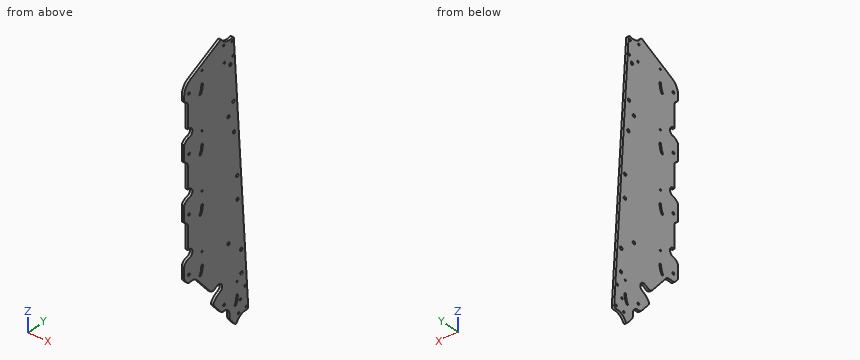
from build123d import *

# Parameters (mm, degrees)
SKETCH_1_R      = 2.5
SKETCH_1_R_2    = 1.6
SKETCH_1_R_3    = 1.3
SKETCH_1_R_4    = 1.9
EXTRUDE_1_DEPTH = 4


with BuildPart() as part:
    # 草图1 → 凸台-拉伸1 (new body)
    with BuildSketch(Plane.ZY):
        with BuildLine():
            Line((79.941847196, 312.779286974), (79.941847196, 310.37938842))
            Line((79.941847196, 310.37938842), (118.048778684, 310.37938842))
            ThreePointArc((118.048778684, 310.37938842), (121.212295154, 309.477639448), (123.424912382, 307.043442935))
            ThreePointArc((123.424912382, 307.043442935), (123.908451597, 306.156590075), (124.459804418, 305.310228312))
            ThreePointArc((124.459804418, 305.310228312), (126.599767036, 303.449448704), (129.355274977, 302.779286974))
            Line((129.355274977, 302.779286974), (135.846674735, 302.779286974))
            ThreePointArc((135.846674735, 302.779286974), (147.714917725, 306.255118752), (155.832977431, 315.5843044))
            Line((155.832977431, 315.5843044), (184.100349844, 377.02653737))
            ThreePointArc((184.100349844, 377.02653737), (184.25423495, 379.122829036), (182.994670387, 380.805569803))
            ThreePointArc((182.994670387, 380.805569803), (175.575423742, 390.035917566), (175.217785471, 401.873004854))
            ThreePointArc((175.217785471, 401.873004854), (174.813539386, 404.446095635), (172.549129806, 405.733208807))
            Line((172.549129806, 405.733208807), (-265.913463366, 435.515010668))
            ThreePointArc((-265.913463366, 435.515010668), (-268.349260645, 434.525893618), (-269.070634733, 431.997835004))
            ThreePointArc((-269.070634733, 431.997835004), (-270.458967767, 420.871071163), (-277.882819523, 412.467573839))
            ThreePointArc((-277.882819523, 412.467573839), (-279.312515533, 410.13392022), (-278.252765969, 407.610648385))
            Line((-278.252765969, 407.610648385), (-268.246230566, 399.190213281))
            ThreePointArc((-268.246230566, 399.190213281), (-265.544431584, 397.566061892), (-262.471282959, 396.863678095))
            Line((-262.471282959, 396.863678095), (-255.629318556, 396.408593428))
            ThreePointArc((-255.629318556, 396.408593428), (-248.6530075, 392.882824378), (-246.344722675, 385.41477346))
            ThreePointArc((-246.344722675, 385.41477346), (-245.547224173, 381.106497376), (-242.780709967, 377.708903254))
            Line((-242.780709967, 377.708903254), (-225.96618646, 363.559589999))
            ThreePointArc((-225.96618646, 363.559589999), (-224.259021966, 363.148943594), (-222.527086507, 363.437804541))
            ThreePointArc((-222.527086507, 363.437804541), (-216.093640019, 369.198004343), (-211.901591148, 376.74756471))
            ThreePointArc((-211.901591148, 376.74756471), (-202.96771311, 381.012048641), (-198.703229179, 372.078170603))
            ThreePointArc((-198.703229179, 372.078170603), (-199.907426668, 369.068297365), (-201.351406018, 366.165823913))
            ThreePointArc((-201.351406018, 366.165823913), (-202.203284687, 360.847165515), (-199.49001514, 356.193995329))
            Line((-199.49001514, 356.193995329), (-166.466058225, 328.404548243))
            ThreePointArc((-166.466058225, 328.404548243), (-163.838636178, 324.972953793), (-162.904676824, 320.753130691))
            Line((-162.904676824, 320.753130691), (-162.904676824, 314.217366152))
            ThreePointArc((-162.904676824, 314.217366152), (-162.15750934, 310.841507671), (-160.055571702, 308.096232111))
            Line((-160.055571702, 308.096232111), (-156.52807865, 305.127869423))
            ThreePointArc((-156.52807865, 305.127869423), (-153.516253341, 303.384762625), (-150.089460052, 302.779286974))
            Line((-150.089460052, 302.779286974), (-132.962822931, 302.779286974))
            ThreePointArc((-132.962822931, 302.779286974), (-131.057359543, 303.089892518), (-129.349178653, 303.989550548))
            ThreePointArc((-129.349178653, 303.989550548), (-127.378799895, 305.843763559), (-125.854682643, 308.079286974))
            ThreePointArc((-125.854682643, 308.079286974), (-124.70730834, 310.334067306), (-124.058152804, 312.779286974))
            ThreePointArc((-124.058152804, 312.779286974), (-117.058152804, 319.779286974), (-110.058152804, 312.779286974))
            Line((-110.058152804, 312.779286974), (-110.058152804, 310.375194841))
            Line((-110.058152804, 310.375194841), (-71.897768127, 310.375194841))
            ThreePointArc((-71.897768127, 310.375194841), (-68.768086545, 309.494285893), (-66.557393134, 307.110225907))
            ThreePointArc((-66.557393134, 307.110225907), (-65.945300527, 306.047683601), (-65.231544729, 305.050584724))
            ThreePointArc((-65.231544729, 305.050584724), (-63.141167069, 303.376870223), (-60.530823557, 302.779286974))
            Line((-60.530823557, 302.779286974), (-36.305637158, 302.779286974))
            ThreePointArc((-36.305637158, 302.779286974), (-33.16644373, 305.003787341), (-30.854682657, 308.079286974))
            ThreePointArc((-30.854682657, 308.079286974), (-29.707305648, 310.334074366), (-29.058150487, 312.779301913))
            ThreePointArc((-29.058150487, 312.779301913), (-22.058145334, 319.779284657), (-15.058155121, 312.779286974))
            Line((-15.058155121, 312.779286974), (-15.058155121, 310.354804619))
            Line((-15.058155121, 310.354804619), (23.075565874, 310.354804619))
            ThreePointArc((23.075565874, 310.354804619), (26.234507213, 309.455891721), (28.446910847, 307.028501158))
            ThreePointArc((28.446910847, 307.028501158), (28.930044794, 306.145924462), (29.48046838, 305.303669209))
            ThreePointArc((29.48046838, 305.303669209), (31.619349297, 303.447603066), (34.37128438, 302.779286974))
            Line((34.37128438, 302.779286974), (58.694362842, 302.779286974))
            ThreePointArc((58.694362842, 302.779286974), (61.833556273, 305.00378734), (64.14531735, 308.079286974))
            ThreePointArc((64.14531735, 308.079286974), (65.292691668, 310.334067319), (65.941847214, 312.779287004))
            ThreePointArc((65.941847214, 312.779287004), (72.94184722, 319.77928698), (79.941847196, 312.779286974))
        make_face()
        with Locations((134.697589837, 398.714435962)):
            Circle(SKETCH_1_R, mode=Mode.SUBTRACT)
        with Locations((-205.302410163, 421.329108832)):
            Circle(SKETCH_1_R, mode=Mode.SUBTRACT)
        with Locations((24.697589837, 406.030947773)):
            Circle(SKETCH_1_R, mode=Mode.SUBTRACT)
        with Locations((54.697589837, 394.714435962)):
            Circle(SKETCH_1_R, mode=Mode.SUBTRACT)
        with Locations((-145.302410163, 394.714435962)):
            Circle(SKETCH_1_R, mode=Mode.SUBTRACT)
        with Locations((-85.302410163, 413.347459584)):
            Circle(SKETCH_1_R, mode=Mode.SUBTRACT)
        with Locations((-229.912547558, 429.226877683)):
            Circle(SKETCH_1_R_2, mode=Mode.SUBTRACT)
        with Locations((-263.830685058, 431.584832)):
            Circle(SKETCH_1_R_2, mode=Mode.SUBTRACT)
        with Locations((-245.82758059, 419.331621378)):
            Circle(SKETCH_1_R_2, mode=Mode.SUBTRACT)
        with Locations((-213.924753581, 412.419296618)):
            Circle(SKETCH_1_R_3, mode=Mode.SUBTRACT)
        with Locations((-265.82758059, 415.709933316)):
            Circle(SKETCH_1_R_2, mode=Mode.SUBTRACT)
        with Locations((145.452321386, 404.165877908)):
            Circle(SKETCH_1_R_2, mode=Mode.SUBTRACT)
        with Locations((172.223627163, 384.384644706)):
            Circle(SKETCH_1_R_2, mode=Mode.SUBTRACT)
        with Locations((169.397149412, 402.539467503)):
            Circle(SKETCH_1_R_2, mode=Mode.SUBTRACT)
        with Locations((144.282792088, 386.203912503)):
            Circle(SKETCH_1_R_2, mode=Mode.SUBTRACT)
        with Locations((-236.412834805, 385.419296624)):
            Circle(SKETCH_1_R_4, mode=Mode.SUBTRACT)
        with Locations((-128.211318153, 339.779286974)):
            Circle(SKETCH_1_R_3, mode=Mode.SUBTRACT)
        with Locations((62, 339.779286968)):
            Circle(SKETCH_1_R_3, mode=Mode.SUBTRACT)
        with Locations((40, 312.779286974)):
            Circle(SKETCH_1_R_4, mode=Mode.SUBTRACT)
        with Locations((-47.3651173, 412.828527404)):
            Circle(SKETCH_1_R, mode=Mode.SUBTRACT)
        with Locations((-55.488081224, 312.779286974)):
            Circle(SKETCH_1_R_4, mode=Mode.SUBTRACT)
        with Locations((-33, 339.779286968)):
            Circle(SKETCH_1_R_3, mode=Mode.SUBTRACT)
        with Locations((-168.130178692, 420.86106375)):
            Circle(SKETCH_1_R, mode=Mode.SUBTRACT)
        with Locations((73.399944092, 404.795991058)):
            Circle(SKETCH_1_R, mode=Mode.SUBTRACT)
        with Locations((157, 339.779286968)):
            Circle(SKETCH_1_R_3, mode=Mode.SUBTRACT)
        with Locations((-150.058152804, 312.779286974)):
            Circle(SKETCH_1_R_4, mode=Mode.SUBTRACT)
        with Locations((135, 312.779286974)):
            Circle(SKETCH_1_R_4, mode=Mode.SUBTRACT)
        with BuildLine():
            ThreePointArc((-235.893747688, 414.018996163), (-243.357483185, 413.10813588), (-250.274012295, 410.158790343))
            ThreePointArc((-250.274012295, 410.158790343), (-250.815185629, 407.961716967), (-248.618112252, 407.420543633))
            ThreePointArc((-248.618112252, 407.420543633), (-242.527853555, 410.017551036), (-235.955759474, 410.819597073))
            ThreePointArc((-235.955759474, 410.819597073), (-234.325054036, 412.388290724), (-235.893747688, 414.018996163))
        make_face(mode=Mode.SUBTRACT)
        with BuildLine():
            ThreePointArc((-54.968994107, 341.378986513), (-62.432729604, 340.468126231), (-69.349258714, 337.518780694))
            ThreePointArc((-69.349258714, 337.518780694), (-69.890432048, 335.321707317), (-67.693358671, 334.780533983))
            ThreePointArc((-67.693358671, 334.780533983), (-61.603099974, 337.377541387), (-55.031005893, 338.179587423))
            ThreePointArc((-55.031005893, 338.179587423), (-53.400300455, 339.748281075), (-54.968994107, 341.378986513))
        make_face(mode=Mode.SUBTRACT)
        with BuildLine():
            ThreePointArc((-150.180312259, 341.378986519), (-157.644047756, 340.468126237), (-164.560576866, 337.5187807))
            ThreePointArc((-164.560576866, 337.5187807), (-165.1017502, 335.321707323), (-162.904676824, 334.780533989))
            ThreePointArc((-162.904676824, 334.780533989), (-156.814418127, 337.377541393), (-150.242324046, 338.179587429))
            ThreePointArc((-150.242324046, 338.179587429), (-148.611618608, 339.748281081), (-150.180312259, 341.378986519))
        make_face(mode=Mode.SUBTRACT)
        with BuildLine():
            ThreePointArc((40.031005893, 341.378986519), (32.567270396, 340.468126237), (25.650741286, 337.5187807))
            ThreePointArc((25.650741286, 337.5187807), (25.109567952, 335.321707323), (27.306641329, 334.780533989))
            ThreePointArc((27.306641329, 334.780533989), (33.396900026, 337.377541393), (39.968994107, 338.179587429))
            ThreePointArc((39.968994107, 338.179587429), (41.599699545, 339.748281081), (40.031005893, 341.378986519))
        make_face(mode=Mode.SUBTRACT)
        with BuildLine():
            ThreePointArc((135.031005893, 341.378986513), (127.567270396, 340.468126231), (120.650741287, 337.518780694))
            ThreePointArc((120.650741287, 337.518780694), (120.109567952, 335.321707317), (122.306641329, 334.780533983))
            ThreePointArc((122.306641329, 334.780533983), (128.396900026, 337.377541387), (134.968994107, 338.179587423))
            ThreePointArc((134.968994107, 338.179587423), (136.599699545, 339.748281075), (135.031005893, 341.378986513))
        make_face(mode=Mode.SUBTRACT)
    extrude(amount=EXTRUDE_1_DEPTH)


solid = part.part
Design review of the part built by this model. Coordinates are the model's own, in mm. Give positions to 0.01 mm unless a question says otherwise; leave off trailing zeros. Loops run counter-clockwise (first coordinate to the right, second up) from the corner with the lowest first, then second, coordinate; pieces in that order, holes last. Notation, with made-up numbers: M 31,47 L 80,47 A30 ccw 80,69 Z; hole C 70,31.25 d3. An arc over 180 degrees is marked long. One line per question, with ' | ' between items. Start each with the question number.
1. Insertion check: P1, Ø1, axis at x = -0.5, z = 64, coming from the +Y side; P2, Ø1.5, axis at x = -3.5, y = 404, coming from the +Z side; P3, Ø1.5, axis at x = -0.5, z = 5.5, coming from the +Y side. Each pin has a flat end and moves straight along its axis. Give the tip position at first contact, or say it passes through.
2. Add section B-B (z = 101). Write out the cut boundary in (x, y), plus the area to 3 significant figures.
3. Add section A-A (x = -1.3). Give the number of separate pieces and of enclosed holes in the cut face, plus the area to 3 significant figures.
4. To check wall thickness, follow L1, parallel to Z at x = -2.9, y = 394.5; L2, parallel to Y at x = -3.1, z = -54; L3, parallel to Y at x = -2.85, z = -204.5. State the ranges of each line that lie inside material, in increasing order.
Worked out:
1) P1: stops at y = 413.14 | P2: stops at z = 175.3 | P3: stops at y = 417.13
2) outline: M -4,310.38 L 0,310.38 L 0,410.59 L -4,410.59 Z | area: 401 mm²
3) separate pieces: 1 | enclosed holes: 32 | area: 42,800 mm²
4) L1: z = -250.39 to -147.79, -142.81 to 52.21, 57.19 to 174.53 | L2: y = 302.78 to 311.6, 313.96 to 338.53, 341.03 to 421.12 | L3: y = 381.37 to 418.96, 423.7 to 431.34
